Can you work these out from the model? Positions are in its coordinate system, mm. Face numbers are marked on the shaded views. A direction names the side the tool comes from. Coordinates: 2 decimals unless noted, no trailing zeros. Write each loop counter-clockwise with the first axis right and the second up, starting at its lowest first coordinate (ties: lowest second). Pieces come first, ordered by that corner, then holes. Notation, with made-up numbers: (-26.5, 31.5) - (18.5, 31.5) arc R26 cw to (18.5, 64.5) - close; hole circle Ø5 at (89.5, 65.25). An arc over 180 degrees is marked (long way). Use one line per item in the form item = value. Start each with the question number.
(1) If we section it at A-A on y = 24.5: Please give me the cut outline in (x, z).
(2) If we section it at D-D on z = 4.5: Please give me the cut outline in (x, y).
(3) If I drill on probe 1 along X at (y, z) = (31, 4.25); probe 2 along Y at (x, z) = (29, 3.5); probe 3 along Y at (x, z) = (16.5, 6.75), over which ranges is the centre line in solid material (lowest first)? Write a range as from..to.
(4) Thinking about a two-plate mould opening in Y: for the marked faces 4, 5 and 6, which applies, pulls with the +Y half, pulls with the -Y half, needs draft (parallel to the pull), parting line crosses it, or undercut?
(5) If we section it at C-C on x = 34: Please give me the cut outline in (y, z), then the cut area to 3 significant figures.
(6) For pin 1 Ø5 at (x, y) = (32, 25.5) entering from -Z; pin 2 Ø1.6 at (x, y) = (17.5, 16) entering from +Z; pin 3 Ø2 at (x, z) = (36, 1.5) entering from +Y; pin 4 Ø6 at (x, z) = (23, 5) entering from +Y, each with a flat end and sliding along its axis, tell me the tip position at first contact or that it passes through.
(7) If we section it at B-B on z = 8: Please give me the cut outline in (x, y).
(8) On a 3-axis mill with a long thin cutter (end or side, diameter ignored), from which of +Z, -Z, +X, -X, +Y, -Y can I reach the whole of each face in a straight line? I mean the marked faces 1, 2 and 3. Say none if no direction works.
```python
from build123d import *

# Parameters (mm, degrees)
F1_DEPTH    = 40
F2_R        = 10
F3_R        = 2
F4_W        = 36
F4_H        = 35.8704487759
F5_DEPTH    = 25
F6_R        = 5
F7_T1_DEPTH = 16.4561700335
F7_T3_DEPTH = 16.4561700335


# Not quite as in the source:
# - a fillet or chamfer that OpenCascade refuses, or shapes differently, is made with other operations: its cross-section is extruded or revolved along the edge and cut away or added


with BuildPart() as f1:
    # F0 (on Right) → F1 (new body)
    with BuildSketch(Plane.YZ):
        Polygon((13, 0), (0, 0), (0, 10), (-2, 10), (-2, -2), (58, -2), (58, 0), (22.1295512241, 0), (22.1295512241, 10), (20.1295512241, 10), (16.4898488815, 0), (15, 0), (18.6397023427, 10), (16.6397023427, 10), align=None)
        with BuildLine():
            Line((22.1295512241, 0), (58, 0))
            ThreePointArc((58, 0), (40.7486885255, 7.4532263127), (22.1295512241, 10))
            Line((22.1295512241, 10), (22.1295512241, 0))
        make_face()
    extrude(amount=F1_DEPTH)

    # F2
    f2_edges = [f1.edges().sort_by_distance(p)[0] for p in [
        (20, 13, 0),
    ]]
    fillet(f2_edges, radius=F2_R)

    # F3
    f3_edges = [f1.edges().sort_by_distance(p)[0] for p in [
        (20, 0, 0),
    ]]
    fillet(f3_edges, radius=F3_R)

    # F4 (on face) → F5 (cut)
    with BuildSketch(Plane.XY.offset(10)):
        with Locations((20, 40.0647756121)):
            Rectangle(F4_W, F4_H)
    extrude(amount=-F5_DEPTH, mode=Mode.SUBTRACT)

    # F6
    f6_edges = [f1.edges().sort_by_distance(p)[0] for p in [
        (2, 22.129551, 4),
        (38, 22.129551, 4),
    ]]
    fillet(f6_edges, radius=F6_R)

    # F7: fillet of radius 5 on 2 edges, made by hand

    # F7_s2 → F7_t1 (cut)
    with BuildSketch(Plane.YZ.offset(-7.2280850168)):
        with BuildLine():
            ThreePointArc((58, -2), (57.132526229, 0.0019440058), (55.4951149029, 1.4438783647))
            ThreePointArc((55.4951149029, 1.4438783647), (56.7550844524, 0.7349972576), (58, 0))
            Line((58, 0), (58, -2))
        make_face()
    extrude(amount=F7_T1_DEPTH, mode=Mode.SUBTRACT)

    # F7_s4 → F7_t3 (cut)
    with BuildSketch(Plane.YZ.offset(30.7719149832)):
        with BuildLine():
            ThreePointArc((58, -2), (57.132526229, 0.0019440058), (55.4951149029, 1.4438783647))
            ThreePointArc((55.4951149029, 1.4438783647), (56.7550844524, 0.7349972576), (58, 0))
            Line((58, 0), (58, -2))
        make_face()
    extrude(amount=F7_T3_DEPTH, mode=Mode.SUBTRACT)


solid = f1.part
```
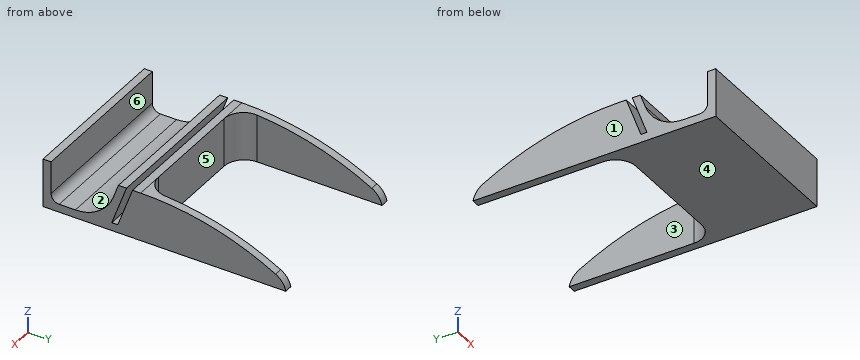
Reported:
q1.outline = (0, -2) - (2.75, -2) - (2.75, 9.96) - (0, 9.96) - close; (37.25, -2) - (40, -2) - (40, 9.96) - (37.25, 9.96) - close
q2.outline = (0, -2) - (40, -2) - (40, 0) - (0, 0) - close; (0, 14.35) - (40, 14.35) - (40, 16.64) - (0, 16.64) - close; (0, 18.13) - (40, 18.13) - (40, 49.19) - (38, 49.19) - (38, 27.13) arc R5 cw to (33, 22.13) - (7, 22.13) arc R5 cw to (2, 27.13) - (2, 49.19) - (0, 49.19) - close
q3.probe_1 = 0..2, 38..40
q3.probe_2 = -2..0, 13.6..16.27, 17.76..22.13
q3.probe_3 = -2..0, 15.46..17.46, 18.95..22.13
q4.face_4 = needs draft
q4.face_5 = pulls with the +Y half
q4.face_6 = undercut
q5.outline = (-2, -2) - (22.23, -2) - (22.23, 10) arc R69.33 ccw to (22.13, 10) - (20.13, 10) - (16.49, 0) - (15, 0) - (18.64, 10) - (16.64, 10) - (15.39, 6.58) arc R10 cw to (6, 0) - (2, 0) arc R2 cw to (0, 2) - (0, 10) - (-2, 10) - close
q5.area = 137 mm2
q6.pin_1 = through
q6.pin_2 = 10
q6.pin_3 = 24.13
q6.pin_4 = 22.13
q7.outline = (0, -2) - (40, -2) - (40, 0) - (0, 0) - close; (0, 15.91) - (40, 15.91) - (40, 17.91) - (0, 17.91) - close; (0, 19.4) - (40, 19.4) - (40, 38.66) - (38, 38.66) - (38, 27.13) arc R5 cw to (33, 22.13) - (7, 22.13) arc R5 cw to (2, 27.13) - (2, 38.66) - (0, 38.66) - close
q8.face_1 = +Z, -Z, -X, +Y, -Y
q8.face_2 = +Z, +X, -X
q8.face_3 = +Z, -Z, +Y
